```python
from build123d import *

# Parameters (mm, degrees)
SKETCH_1_W      = 12.7
SKETCH_1_H      = 6.7
EXTRUDE_1_DEPTH = 6.3
SKETCH_2_W      = 3.9
SKETCH_2_H      = 3.9
EXTRUDE_2_DEPTH = 5
SKETCH_3_W      = 0.8
SKETCH_3_H      = 1.3
EXTRUDE_3_DEPTH = 6.9


with BuildPart() as part:
    # 草图1 → 凸台-拉伸1 (new body)
    with BuildSketch(Plane(origin=(0, 0, 0), x_dir=(1, 0, 0), z_dir=(0, 1, 0))):
        Rectangle(SKETCH_1_W, SKETCH_1_H)
    extrude(amount=EXTRUDE_1_DEPTH)

    # 草图2 → 凸台-拉伸2 (add)
    with BuildSketch(Plane(origin=(0, 6.3, 0), x_dir=(1, 0, 0), z_dir=(0, 1, 0))):
        Rectangle(SKETCH_2_W, SKETCH_2_H)
    extrude(amount=EXTRUDE_2_DEPTH)

    # 草图3 → 凸台-拉伸3 (add)
    with BuildSketch(Plane.XZ):
        Rectangle(SKETCH_3_W, SKETCH_3_H)
        with Locations((4.8, 0)):
            Rectangle(SKETCH_3_W, SKETCH_3_H)
        with Locations((-4.8, 0)):
            Rectangle(SKETCH_3_W, SKETCH_3_H)
    extrude(amount=EXTRUDE_3_DEPTH)


solid = part.part
```
CAD build for the part. Positions are in the model's coordinates, mm. A direction names the side the tool comes from. Coordinates: 2 decimals unless noted, no trailing zeros. Write each loop counter-clockwise with the first axis right and the second up, starting at its lowest first coordinate (ties: lowest second). Pieces come first, ordered by that corner, then holes.
(1) Cut at C-C, the plane z = 0. List the corners of the cut face in (x, y).
(2) Drill centre lines: probe 1 along X at (y, z) = (-3.75, -0.5); probe 2 along Y at (x, z) = (2.75, 0.75); probe 3 along Y at (x, z) = (0.5, 0.75). Where is each one in solid material? Low to high.
(3) Cut at A-A, the plane y = -0.75. List the corners of the cut face in (x, z).
(4) 3-axis set-ups, long thin cutter, end or side, ignore diameter. For faces 1 (the face through (-5, -3, -0.65)), 2 (the face through (0, 9, -1.95)), 3 (the face through (1.95, 9, 0)), 4 (the face through (-5.2, -3, 0)): which of +Z, -Z, +X, -X, +Y, -Y reach the whole face in a straight line?
(5) Cut at B-B, the plane x = -1.75. List the corners of the cut face in (y, z), and give its area (3 significant figures).
(6) Two-plate mould, pull along X, no slides. Class faces 5 (the face through (6.35, 3, 0)), 6 (the face through (5, -3, 0.65)), 7 (the face through (-0.4, -3, 0)): +X half, -X half, draft (parallel to the pull), parting line (faces both ways), or undercut.
(7) Flat gauge pins, fed straight in: pin 1 (0.6 mm diameter, centred on x = 0, y = -4, fed in from +Z); pin 2 (1 mm diameter, centred on y = -3.5, z = 0, fed in from -X); pin 3 (0.9 mm diameter, centred on x = 5, y = -4, fed in from -Z). Where does each tip first touch, or does it go through?
(8) Cut at D-D, the plane x = -4.75. List the corners of the cut face in (y, z), and give its area (3 significant figures).
Geometry says:
1. outline: (-6.35, 0) - (-5.2, 0) - (-5.2, -6.9) - (-4.4, -6.9) - (-4.4, 0) - (-0.4, 0) - (-0.4, -6.9) - (0.4, -6.9) - (0.4, 0) - (4.4, 0) - (4.4, -6.9) - (5.2, -6.9) - (5.2, 0) - (6.35, 0) - (6.35, 6.3) - (1.95, 6.3) - (1.95, 11.3) - (-1.95, 11.3) - (-1.95, 6.3) - (-6.35, 6.3) - close
2. probe 1: x = -5.2 to -4.4, -0.4 to 0.4, 4.4 to 5.2
2. probe 2: y = 0 to 6.3
2. probe 3: y = 0 to 11.3
3. outline: (-5.2, -0.65) - (-4.4, -0.65) - (-4.4, 0.65) - (-5.2, 0.65) - close; (-0.4, -0.65) - (0.4, -0.65) - (0.4, 0.65) - (-0.4, 0.65) - close; (4.4, -0.65) - (5.2, -0.65) - (5.2, 0.65) - (4.4, 0.65) - close
4. face 1: -Z, +X, -X, -Y
4. face 2: -Z, +X, -X, +Y
4. face 3: +Z, -Z, +X, +Y
4. face 4: +Z, -Z, -X, -Y
5. outline: (0, -3.35) - (6.3, -3.35) - (6.3, -1.95) - (11.3, -1.95) - (11.3, 1.95) - (6.3, 1.95) - (6.3, 3.35) - (0, 3.35) - close
5. area: 61.7 mm2
6. face 5: +X half
6. face 6: draft
6. face 7: undercut
7. pin 1: stops at z = 0.65
7. pin 2: stops at x = -5.2
7. pin 3: stops at z = -0.65
8. outline: (-6.9, -0.65) - (0, -0.65) - (0, -3.35) - (6.3, -3.35) - (6.3, 3.35) - (0, 3.35) - (0, 0.65) - (-6.9, 0.65) - close
8. area: 51.2 mm2
